from build123d import *

# Parameters (mm, degrees)
ESBO_O1_R                = 25
ESBO_O1_R_2              = 3.1
RESSALTO_EXTRUS_O1_DEPTH = 40
ESBO_O3_R                = 21
CORTE_EXTRUS_O1_DEPTH    = 7.7
CORTE_EXTRUS_O2_START    = -7.7
ESBO_O4_R                = 21
CORTE_EXTRUS_O2_DEPTH    = 7.7
FILETE1_R                = 1
ESBO_O11_R               = 22.5
ESBO_O11_R_2             = 21
CORTE_EXTRUS_O3_DEPTH    = 2
CORTE_EXTRUS_O4_START    = -2
ESBO_O12_R               = 22.5
ESBO_O12_R_2             = 21
CORTE_EXTRUS_O4_DEPTH    = 2


with BuildPart() as part:
    # Esboço1 → Ressalto-extrusão1 (new, symmetric)
    with BuildSketch(Plane.XY):
        Circle(ESBO_O1_R)
        Circle(ESBO_O1_R_2, mode=Mode.SUBTRACT)
    extrude(amount=RESSALTO_EXTRUS_O1_DEPTH, both=True)

    # Esboço3 → Corte-extrusão1 (cut)
    with BuildSketch(Plane.XY.offset(40)):
        Circle(ESBO_O3_R)
    extrude(amount=-CORTE_EXTRUS_O1_DEPTH, mode=Mode.SUBTRACT)

    # Esboço4 → Corte-extrusão2 (cut)
    with BuildSketch(Plane(origin=(0, 0, -40), x_dir=(-1, 0, 0), z_dir=(0, 0, -1)).offset(CORTE_EXTRUS_O2_START)):
        with Locations(Location((0, 0, 0), (0, 0, 180))):
            Circle(ESBO_O4_R)
    extrude(amount=CORTE_EXTRUS_O2_DEPTH, mode=Mode.SUBTRACT)

    # Filete1
    filete1_edges = [part.edges().sort_by_distance(p)[0] for p in [
        (-21, 0, 32.3),
        (-3.1, 0, 32.3),
        (-21, 0, -32.3),
        (-3.1, 0, -32.3),
    ]]
    fillet(filete1_edges, radius=FILETE1_R)

    # Esboço11 → Corte-extrusão3 (cut)
    with BuildSketch(Plane.XY.offset(40)):
        Circle(ESBO_O11_R)
        Circle(ESBO_O11_R_2, mode=Mode.SUBTRACT)
    extrude(amount=-CORTE_EXTRUS_O3_DEPTH, mode=Mode.SUBTRACT)

    # Esboço12 → Corte-extrusão4 (cut)
    with BuildSketch(Plane(origin=(0, 0, -40), x_dir=(-1, 0, 0), z_dir=(0, 0, -1)).offset(CORTE_EXTRUS_O4_START)):
        with Locations(Location((0, 0, 0), (0, 0, 180))):
            Circle(ESBO_O12_R)
        Circle(ESBO_O12_R_2, mode=Mode.SUBTRACT)
    extrude(amount=CORTE_EXTRUS_O4_DEPTH, mode=Mode.SUBTRACT)


solid = part.part
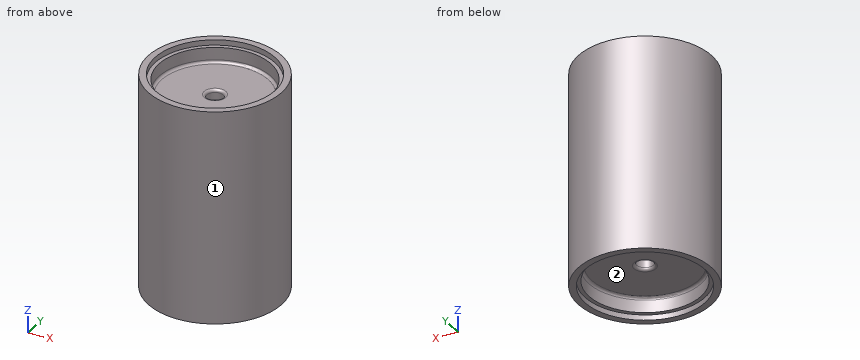
For this review, take the finished solid that the model builds, in its own axes (mm). Face numbers are marked on the shaded views. Give positions to 0.01 mm unless a question says otherwise; leave off trailing zeros. Order: outer loops, then holes, each group sorted by start corner. A loop starts at its lowest first (then second) coordinate and runs counter-clockwise, first axis right, second up. Notation, with made-up numbers: (40.5, 76.25) -> (88.5, 76.25) arc R15 cw to (88.5, 83.25) -> close; hole circle Ø2 at (-34.5, 49). An arc over 180 degrees is marked (long way). Write item = value, one per line.
1) We need section C-C, the plane z = -19. Give the boundary of the cut face in (x, y).
Findings:
outline = circle Ø50 at (0, 0); hole circle Ø6.2 at (0, 0)
2) Draft analysis for pull direction X (two halves, no side actions). For the marked faces 1 and 2, state which applies: pulls with the +X half, pulls with the -X half, needs draft (parallel to the pull), parting line crosses it, or undercut.
Findings:
face_1 = parting line crosses it
face_2 = undercut
3) Insertion check: pin 1 (1 mm diameter, centred on x = 17.5, y = 8.5, fed in from -Z); pin 2 (6 mm diameter, centred on y = -11.5, z = -5.5, fed in from +X); pin 3 (4 mm diameter, centred on x = -11.5, z = -30, fed in from +Y). Each pin has a flat end and moves straight along its axis. Give the tip position at first contact, or say it passes through.
Findings:
pin_1 = -32.3
pin_2 = 23.51
pin_3 = 23.12
4) To check wall thickness, follow L1, parallel to Y at x = 0, z = -34; L2, parallel to Y at x = 0, z = 38.8; L3, parallel to Z at x = 5, y = -6. State the ranges of each line that lie inside material, in increasing order. Write a range as from..to.
Findings:
L1 = -25..-21, 21..25
L2 = -25..-22.5, 22.5..25
L3 = -32.3..32.3
5) We need section D-D, the plane z = -34.5. Give the boundary of the cut face in (x, y).
Findings:
outline = circle Ø50 at (0, 0); hole circle Ø42 at (0, 0)
